from build123d import *

# Parameters (mm, degrees)
F0_W     = 17
F0_H     = 64.5
F0_H_2   = 12
F0_R     = 5
F1_DEPTH = 2
F2_R     = 8
F3_SIZE  = 1.99999
F0_R_2   = 2.2
F4_DEPTH = 1
F5_DEPTH = 3
F6_R     = 8
F7_SIZE  = 0.99999


# Not quite as in the source:
# - a fillet or chamfer is up to 0.001 mm smaller than in the source, because OpenCascade refuses the exact size


with BuildPart() as f1:
    # F0 (on Top) → F1 (new body)
    with BuildSketch(Plane.XY):
        with Locations((0, 6)):
            Rectangle(F0_W, F0_H)
        with Locations((0, -32.25)):
            Rectangle(F0_W, F0_H_2)
        with Locations((0, -33.05)):
            Circle(F0_R, mode=Mode.SUBTRACT)
    extrude(amount=F1_DEPTH)

    # F2
    f2_edges = [f1.edges().sort_by_distance(p)[0] for p in [
        (8.5, -38.25, 1),
        (-8.5, -38.25, 1),
    ]]
    fillet(f2_edges, radius=F2_R)

    # F3 (size 2 in the source; OpenCascade refuses exactly that, so slightly less here)
    f3_edges = [f1.edges().sort_by_distance(p)[0] for p in [
        (0, 38.25, 0),
    ]]
    chamfer(f3_edges, length=F3_SIZE)

    # F0 (on Top) → F4 (join)
    with BuildSketch(Plane.XY):
        with Locations((0, -33.05)):
            Circle(F0_R)
        with Locations((0, -33.05)):
            Circle(F0_R_2, mode=Mode.SUBTRACT)
    extrude(amount=F4_DEPTH)

    # F0 (on Top) → F5 (join)
    with BuildSketch(Plane.XY):
        with Locations((0, -32.25)):
            Rectangle(F0_W, F0_H_2)
        with Locations((0, -33.05)):
            Circle(F0_R, mode=Mode.SUBTRACT)
    extrude(amount=F5_DEPTH)

    # F6
    f6_edges = [f1.edges().sort_by_distance(p)[0] for p in [
        (8.5, -38.25, 1.5),
        (-8.5, -38.25, 1.5),
    ]]
    fillet(f6_edges, radius=F6_R)

    # F7 (size 1 in the source; OpenCascade refuses exactly that, so slightly less here)
    f7_edges = [f1.edges().sort_by_distance(p)[0] for p in [
        (0, -26.25, 3),
    ]]
    chamfer(f7_edges, length=F7_SIZE)


solid = f1.part
For this review, take the finished solid that the model builds, in its own axes (mm). A direction names the side the tool comes from. Coordinates: 2 decimals unless noted, no trailing zeros. Loops run counter-clockwise (first coordinate to the right, second up) from the corner with the lowest first, then second, coordinate; pieces in that order, holes last. Notation, with made-up numbers: (41.25, 79) -> (81.25, 79) arc R6 cw to (81.25, 85) -> close; hole circle Ø7 at (89, -32). An arc over 180 degrees is marked (long way). Write each question's results on one line, items separated by ' | '.
Q1. Add section A-A, the plane y = -33.05. State the section outline as (x, z) points, then the cut area to 3 significant figures.
Taken from the geometry:
outline: (-7.99, 0) -> (-2.2, 0) -> (-2.2, 1) -> (-5, 1) -> (-5, 3) -> (-7.99, 3) -> close; (2.2, 0) -> (7.99, 0) -> (7.99, 3) -> (5, 3) -> (5, 1) -> (2.2, 1) -> close | area: 23.6 mm²
Q2. Add section C-C, the plane y = 15.5. State the section outline as (x, z) points, then the cut area to 3 significant figures.
Taken from the geometry:
outline: (-8.5, 0) -> (8.5, 0) -> (8.5, 2) -> (-8.5, 2) -> close | area: 34.0 mm²
Q3. Mouldability with a two-part tool opening along Y and no side actions: class faces 1 (the flat face through (1, -35.2, 1)), 2 (the cylindrical face through (-6.219, -35.844, 1.521)), 3 (the flat face through (-8.5, 4, 1)) as +Y half, -Y half, draft (parallel to the pull), parting line (faces both ways), or undercut.
Taken from the geometry:
face 1: undercut | face 2: -Y half | face 3: draft
Q4. For pin 1 Ø2.5 at (x, y) = (0, -33.05) entering from +Z; pin 2 Ø5 at (x, y) = (-1, -18.5) entering from +Z; pin 3 Ø5 at (x, y) = (0.5, -32) entering from +Z; pin 4 Ø8 at (x, y) = (0, -33.05) entering from -Z, all flat-tipped, find the tip position at first contact; note any pin that passes through.
Taken from the geometry:
pin 1: through | pin 2: z = 2 | pin 3: z = 1 | pin 4: z = 0
Q5. To check wall thickness, follow line 1 along Z through (x, y) = (6.25, 2.5); line 2 along Y through (x, z) = (0, 0.3); line 3 along Y through (x, z) = (0, 0.75). State the ranges of each line that lie inside material, in increasing order. Write a range as [from, to].
Taken from the geometry:
line 1: [0, 2] | line 2: [-38.25, -35.25], [-30.85, 36.55] | line 3: [-38.25, -35.25], [-30.85, 37]
Q6. Machinability: for faces 4 (the flat face through (0, 6, 2)), 5 (the flat face through (-0.12, 37.26, 1.01)), 6 (the cylindrical face through (-0.7, -28.1, 2)), which of the approach directions +Z, -Z, +X, -X, +Y, -Y give a long, thin tool a straight path to every point of the face, cutting with its end or side? Answer none if there is none.
Taken from the geometry:
face 4: +Z, +X, -X, +Y | face 5: -Z, +X, -X, +Y | face 6: +Z
